```python
from build123d import *

# Parameters (mm, degrees)
BOSS_EXTRUDE1_DEPTH     = 220
CUT_EXTRUDE1_DEPTH      = 10
SKETCH3_R               = 1.5
SKETCH3_W               = 30
SKETCH3_H               = 35
SKETCH3_W_2             = 50
CUT_EXTRUDE2_DEPTH      = 274
SKETCH5_R               = 1.5
CUT_EXTRUDE3_DEPTH      = 10
SKETCH6_R               = 1.5
CUT_EXTRUDE4_DEPTH      = 10
SKETCH7_R               = 1.5
CUT_EXTRUDE5_DEPTH      = 77.5
CUT_EXTRUDE5_DEPTH_BACK = 2.5
SKETCH8_R               = 1.5
CUT_EXTRUDE6_DEPTH      = 79
SKETCH9_R               = 1.5
CUT_EXTRUDE7_DEPTH      = 274


with BuildPart() as part:
    # Sketch1 → Boss-Extrude1 (new body)
    with BuildSketch(Plane(origin=(0, 0, 0), x_dir=(0, 0, -1), z_dir=(1, 0, 0))):
        with BuildLine():
            Line((-125, 39), (125, 39))
            ThreePointArc((125, 39), (133.131727984, 35.631727984), (136.5, 27.5))
            Line((136.5, 27.5), (136.5, -27.5))
            ThreePointArc((136.5, -27.5), (133.131727984, -35.631727984), (125, -39))
            Line((125, -39), (-125, -39))
            ThreePointArc((-125, -39), (-133.131727984, -35.631727984), (-136.5, -27.5))
            Line((-136.5, -27.5), (-136.5, 27.5))
            ThreePointArc((-136.5, 27.5), (-133.131727984, 35.631727984), (-125, 39))
        make_face()
        with BuildLine():
            Line((-125, 37.5), (125, 37.5))
            ThreePointArc((125, 37.5), (132.071067812, 34.571067812), (135, 27.5))
            Line((135, 27.5), (135, -27.5))
            ThreePointArc((135, -27.5), (132.071067812, -34.571067812), (125, -37.5))
            Line((125, -37.5), (-125, -37.5))
            ThreePointArc((-125, -37.5), (-132.071067812, -34.571067812), (-135, -27.5))
            Line((-135, -27.5), (-135, 27.5))
            ThreePointArc((-135, 27.5), (-132.071067812, 34.571067812), (-125, 37.5))
        make_face(mode=Mode.SUBTRACT)
    extrude(amount=BOSS_EXTRUDE1_DEPTH)

    # Sketch2 → Cut-Extrude1 (cut)
    with BuildSketch(Plane(origin=(0, 39, 0), x_dir=(1, 0, 0), z_dir=(0, 1, 0))):
        with BuildLine():
            Line((15, 90), (0, 90))
            Line((0, 90), (0, -90))
            Line((0, -90), (15, -90))
            ThreePointArc((15, -90), (20.857864376, -104.142135624), (35, -110))
            Line((35, -110), (185, -110))
            ThreePointArc((185, -110), (199.142135624, -104.142135624), (205, -90))
            Line((205, -90), (220, -90))
            Line((220, -90), (220, 90))
            Line((220, 90), (205, 90))
            ThreePointArc((205, 90), (199.142135624, 104.142135624), (185, 110))
            Line((185, 110), (35, 110))
            ThreePointArc((35, 110), (20.857864376, 104.142135624), (15, 90))
        make_face()
    extrude(amount=-CUT_EXTRUDE1_DEPTH, mode=Mode.SUBTRACT)

    # Sketch3 → Cut-Extrude2 (cut, through all)
    with BuildSketch(Plane.XY.offset(136.5)):
        with Locations((77.5, 17.5)):
            Circle(SKETCH3_R)
        with Locations((77.5, -17.5)):
            Circle(SKETCH3_R)
        with Locations((142.5, 17.5)):
            Circle(SKETCH3_R)
        with Locations((142.5, -17.5)):
            Circle(SKETCH3_R)
        with Locations((32.5, 17.5)):
            Circle(SKETCH3_R)
        with Locations((32.5, -17.5)):
            Circle(SKETCH3_R)
        with Locations((187.5, 17.5)):
            Circle(SKETCH3_R)
        with Locations((187.5, -17.5)):
            Circle(SKETCH3_R)
        with Locations((55, 0)):
            Rectangle(SKETCH3_W, SKETCH3_H)
        with Locations((165, 0)):
            Rectangle(SKETCH3_W, SKETCH3_H)
        with Locations((110, 0)):
            Rectangle(SKETCH3_W_2, SKETCH3_H)
    extrude(amount=-CUT_EXTRUDE2_DEPTH, mode=Mode.SUBTRACT)

    # Sketch5 → Cut-Extrude3 (cut)
    with BuildSketch(Plane(origin=(0, -37.5, 0), x_dir=(1, 0, 0), z_dir=(0, 1, 0))):
        with Locations((79, -55)):
            Circle(SKETCH5_R)
        with Locations((79, -10)):
            Circle(SKETCH5_R)
    extrude(amount=-CUT_EXTRUDE3_DEPTH, mode=Mode.SUBTRACT)

    # Sketch6 → Cut-Extrude4 (cut)
    with BuildSketch(Plane(origin=(0, -37.5, 0), x_dir=(1, 0, 0), z_dir=(0, 1, 0))):
        with Locations((110, -77.5)):
            Circle(SKETCH6_R)
        with Locations((140, -77.5)):
            Circle(SKETCH6_R)
        with Locations((170, -77.5)):
            Circle(SKETCH6_R)
        with Locations((80, -77.5)):
            Circle(SKETCH6_R)
        with Locations((50, -77.5)):
            Circle(SKETCH6_R)
        with Locations((110, 77.5)):
            Circle(SKETCH6_R)
        with Locations((140, 77.5)):
            Circle(SKETCH6_R)
        with Locations((170, 77.5)):
            Circle(SKETCH6_R)
        with Locations((80, 77.5)):
            Circle(SKETCH6_R)
        with Locations((50, 77.5)):
            Circle(SKETCH6_R)
    extrude(amount=-CUT_EXTRUDE4_DEPTH, mode=Mode.SUBTRACT)

    # Sketch7 → Cut-Extrude5 (cut, two sides)
    with BuildSketch(Plane(origin=(0, -37.5, 0), x_dir=(1, 0, 0), z_dir=(0, 1, 0))) as cut_extrude5_sk:
        with Locations((7.5, 10)):
            Circle(SKETCH7_R)
        with Locations((7.5, -10)):
            Circle(SKETCH7_R)
        with Locations((7.5, -40)):
            Circle(SKETCH7_R)
        with Locations((7.5, -70)):
            Circle(SKETCH7_R)
        with Locations((7.5, -100)):
            Circle(SKETCH7_R)
        with Locations((7.5, 40)):
            Circle(SKETCH7_R)
        with Locations((7.5, 70)):
            Circle(SKETCH7_R)
        with Locations((7.5, 100)):
            Circle(SKETCH7_R)
    extrude(amount=CUT_EXTRUDE5_DEPTH, mode=Mode.SUBTRACT)
    extrude(cut_extrude5_sk.sketch, amount=-CUT_EXTRUDE5_DEPTH_BACK, mode=Mode.SUBTRACT)

    # Sketch8 → Cut-Extrude6 (cut, through all)
    with BuildSketch(Plane.XZ.offset(39)):
        with Locations((212.5, 10)):
            Circle(SKETCH8_R)
        with Locations((212.5, -10)):
            Circle(SKETCH8_R)
        with Locations((212.5, -40)):
            Circle(SKETCH8_R)
        with Locations((212.5, -70)):
            Circle(SKETCH8_R)
        with Locations((212.5, -100)):
            Circle(SKETCH8_R)
        with Locations((212.5, 40)):
            Circle(SKETCH8_R)
        with Locations((212.5, 70)):
            Circle(SKETCH8_R)
        with Locations((212.5, 100)):
            Circle(SKETCH8_R)
    extrude(amount=-CUT_EXTRUDE6_DEPTH, mode=Mode.SUBTRACT)

    # Sketch9 → Cut-Extrude7 (cut, through all)
    with BuildSketch(Plane(origin=(0, 0, -136.5), x_dir=(-1, 0, 0), z_dir=(0, 0, -1))):
        with Locations((-7.5, 0)):
            Circle(SKETCH9_R)
        with Locations((-7.5, 15)):
            Circle(SKETCH9_R)
        with Locations((-7.5, -15)):
            Circle(SKETCH9_R)
        with Locations((-212.5, 0)):
            Circle(SKETCH9_R)
        with Locations((-212.5, 15)):
            Circle(SKETCH9_R)
        with Locations((-212.5, -15)):
            Circle(SKETCH9_R)
    extrude(amount=-CUT_EXTRUDE7_DEPTH, mode=Mode.SUBTRACT)


solid = part.part
```
Input: part model. Units: mm. Frame: model coordinates. A direction names the side the tool comes from. Give positions to 0.01 mm unless a question says otherwise; leave off trailing zeros. Order: outer loops, then holes, each group sorted by start corner. A loop starts at its lowest first (then second) coordinate and runs counter-clockwise, first axis right, second up. Notation, with made-up numbers: M 67,6 L 79,6 A15 ccw 79,18 Z; hole C 66.5,23.25 d7. An arc over 180 degrees is marked long. One line per question, with ' | ' between items. Start each with the question number.
1. Section query B-B (x = 103.5). Return the cut outline in (y, z).
2. Section query A-A (y = 7.5). Count the separate pieces of the cut face and the enclosed holes in it, and give its area (3 significant figures).
3. Section query D-D (z = 46.5). Return the cut outline in (x, y), and give its area (3 significant figures).
4. Material intervals for probe 1 along X at (y, z) = (-38.4, 100); probe 2 along Z at (x, y) = (131.5, 22.5); probe 3 along Z at (x, y) = (188, 28.5), sorted ascending. Write a range as [from, to].
5. Pull-direction query (Y, two-part tool) for faces 1 (the face through (108, -39, -2)), 2 (the face through (108.46, 34.65, -131.99)), 3 (the face through (21.014, 38.26, -104.297)), 4 (the face through (108.46, 34.49, 132.15)); classes: released by +Y, released by -Y, zero draft, split by the parting line, or undercut.
6. First-contact query: pin 1 Ø2.5 at (x, y) = (77.5, 17.5) entering from +Z; pin 2 Ø0.8 at (x, z) = (60.5, -136) entering from +Y; pin 3 Ø4 at (x, z) = (7.5, -70) entering from +Y. Flat tips, straight axial feed; report the tip coordinate or a pass-through.
7. Section query C-C (z = -105.5). Return the cut outline in (x, y), and give its area (3 significant figures).
8. Access query for faces 5 (the face through (108, 39, -115)), 6 (the face through (108.46, -34.49, -132.15)), 7 (the face through (199.297, 38.26, -103.986)). Directions: +Z, -Z, +X, -X, +Y, -Y. A direction counts if a zero-diameter tool reaches every point of the face in a straight line with its end or side. Return the directions, or none.
Here are the results:
1) outline: M -39,-125 A11.5 ccw -27.5,-136.5 L -17.5,-136.5 L -17.5,-135 L -27.5,-135 A10 cw -37.5,-125 L -37.5,125 A10 cw -27.5,135 L -17.5,135 L -17.5,136.5 L -27.5,136.5 A11.5 ccw -39,125 Z; M 17.5,-136.5 L 27.5,-136.5 A11.5 ccw 39,-125 L 39,-110 L 37.5,-110 L 37.5,-125 A10 cw 27.5,-135 L 17.5,-135 Z; M 17.5,135 L 27.5,135 A10 cw 37.5,125 L 37.5,110 L 39,110 L 39,125 A11.5 ccw 27.5,136.5 L 17.5,136.5 Z
2) separate pieces: 8 | enclosed holes: 0 | area: 330 mm²
3) outline: M 0,-39 L 220,-39 L 220,-37.5 L 0,-37.5 Z | area: 330 mm²
4) probe 1: [0, 6], [9, 211], [214, 220] | probe 2: [-136.5, -135], [135, 136.5] | probe 3: [-136.46, -134.95], [134.95, 136.46]
5) face 1: released by -Y | face 2: undercut | face 3: zero draft | face 4: undercut
6) pin 1: through | pin 2: y = 31.96 | pin 3: y = -37.5
7) outline: M 0,-39 L 220,-39 L 220,-37.5 L 0,-37.5 Z; M 0,37.5 L 22.36,37.5 L 22.36,39 L 0,39 Z; M 197.64,37.5 L 220,37.5 L 220,39 L 197.64,39 Z | area: 397 mm²
8) face 5: +Z, -Z, +X, -X, +Y | face 6: +X, -X | face 7: +Y
